Part model, mm, in its own coordinate system. Round coordinates to 2 decimals unless told otherwise and drop trailing zeros. Loops run counter-clockwise (first coordinate to the right, second up) from the corner with the lowest first, then second, coordinate; pieces in that order, holes last.
1) Band-saw the part on B-B, the plane x = -738.5. Write the cut outline in (y, z), then the cut area to 3 significant figures.
2) Band-saw the part on A-A, the plane y = 9.25. Write the cut outline in (x, z), then the cut area to 3 significant figures.
3) Probe line 1 (Z direction, x = -313.5, y = 19.5); line 2 (Z direction, x = -723, y = 10); line 3 (Z direction, x = -558, y = 2.75). List the from-to ranges inside material, lowest first.
4) Drop flat-ended pins along their axis: P1, Ø5, axis at x = -136, z = 3, coming from the -Y side; P2, Ø0.6, axis at x = -16.5, z = 15, coming from the -Y side; P3, Ø1.3, axis at x = -177, z = 12.5, coming from the -Y side; P4, Ø1.5, axis at x = 151, z = 7, coming from the +Y side. Give the stop position or say it passes through.
5) Band-saw the part on C-C, the plane z = 7.62. Write the cut outline in (x, y).
from build123d import *

# Parameters (mm, degrees)
BOSS_EXTRUDE1_DEPTH       = 934.24375
CUT_TOP_RIGHT_FRONT_DEPTH = 22.844
CUT_TOP_LEFT_FRONT_DEPTH  = 22.844


with BuildPart() as part:
    # Sketch1 → Boss-Extrude1 (new body, symmetric)
    with BuildSketch(Plane(origin=(0, 0, 0), x_dir=(0, 0, -1), z_dir=(1, 0, 0))):
        with BuildLine():
            Line((0, 0), (0, 21.844))
            Line((0, 21.844), (-5.08, 21.844))
            Line((-5.08, 21.844), (-5.08, 20.066))
            ThreePointArc((-5.08, 20.066), (-7.62, 17.526), (-10.16, 20.066))
            Line((-10.16, 20.066), (-10.16, 21.844))
            Line((-10.16, 21.844), (-15.24, 21.844))
            Line((-15.24, 21.844), (-15.24, 3.048))
            Line((-15.24, 3.048), (-13.97, 3.048))
            Line((-13.97, 3.048), (-13.97, 20.574))
            Line((-13.97, 20.574), (-11.43, 20.574))
            Line((-11.43, 20.574), (-11.43, 20.066))
            ThreePointArc((-11.43, 20.066), (-7.62, 16.256), (-3.81, 20.066))
            Line((-3.81, 20.066), (-3.81, 20.574))
            Line((-3.81, 20.574), (-1.27, 20.574))
            Line((-1.27, 20.574), (-1.27, 0))
            Line((-1.27, 0), (0, 0))
        make_face()
    extrude(amount=BOSS_EXTRUDE1_DEPTH, both=True)

    # Sketch2 → Cut-Top-Right-Front (cut, through all)
    with BuildSketch(Plane(origin=(0, 21.844, 0), x_dir=(1, 0, 0), z_dir=(0, 1, 0))):
        Polygon((934.24375, 0), (919.00375, -15.24), (934.24375, -15.24), align=None)
    extrude(amount=-CUT_TOP_RIGHT_FRONT_DEPTH, mode=Mode.SUBTRACT)

    # Sketch4 → Cut-Top-Left-Front (cut, through all)
    with BuildSketch(Plane(origin=(0, 21.844, 0), x_dir=(1, 0, 0), z_dir=(0, 1, 0))):
        Polygon((-934.24375, 0), (-919.00375, -15.24), (-934.24375, -15.24), align=None)
    extrude(amount=-CUT_TOP_LEFT_FRONT_DEPTH, mode=Mode.SUBTRACT)


solid = part.part
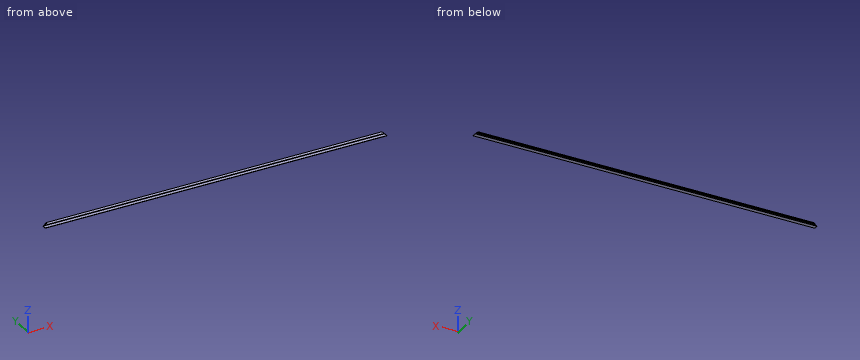
Reported:
1. outline: (0, 0) - (21.84, 0) - (21.84, 5.08) - (20.07, 5.08) arc R2.54 cw to (20.07, 10.16) - (21.84, 10.16) - (21.84, 15.24) - (3.05, 15.24) - (3.05, 13.97) - (20.57, 13.97) - (20.57, 11.43) - (20.07, 11.43) arc R3.81 ccw to (20.07, 3.81) - (20.57, 3.81) - (20.57, 1.27) - (0, 1.27) - close
1. area: 75.2 mm2
2. outline: (-934.24, 0) - (934.24, 0) - (932.97, 1.27) - (-932.97, 1.27) - close; (-920.27, 13.97) - (920.27, 13.97) - (919, 15.24) - (-919, 15.24) - close
2. area: 4,710 mm2
3. line 1: z = 0 to 1.27, 3.85 to 5.14, 10.1 to 11.39, 13.97 to 15.24
3. line 2: z = 0 to 1.27, 13.97 to 15.24
3. line 3: z = 0 to 1.27
4. P1: stops at y = 0
4. P2: stops at y = 3.05
4. P3: stops at y = 20.57
4. P4: stops at y = 17.93
5. outline: (-926.62, 16.26) - (926.62, 16.26) - (926.62, 17.53) - (-926.62, 17.53) - close
